Can you work these out from the model? Positions are in its coordinate system, mm. A direction names the side the tool comes from. Give positions to 0.01 mm unless a question says otherwise; leave off trailing zeros. Order: outer loops, then holes, each group sorted by start corner. A loop starts at its lowest first (then second) coordinate and runs counter-clockwise, first axis right, second up. Notation, with made-up numbers: M 23,35.5 L 48,35.5 A23 ccw 48,58.5 Z; hole C -27,9 d7. An arc over 180 degrees is marked long. Answer as a JSON object with one key per item and string values.
```python
from build123d import *

# Parameters (mm, degrees)
SKETCH1_W           = 32
SKETCH1_H           = 22
SKETCH1_W_2         = 30
SKETCH1_H_2         = 20
SKETCH3_W           = 30
SKETCH3_H           = 22
SKETCH3_W_2         = 28
SKETCH3_H_2         = 20
EXTRUDE_THIN1_DEPTH = 150


with BuildPart() as part:
    # Sweep-Thin1: sweep along a path in Sketch2
    with BuildLine(Plane(origin=(0, 0, 0), x_dir=(0, 0, -1), z_dir=(1, 0, 0))) as sweep_thin1_path:
        Line((0, 0), (0, -200))
        Line((0, -200), (428, -200))
        Line((428, -200), (428, 0))
    # Sketch1 → Sweep-Thin1 (sweep)
    with BuildSketch(Plane(origin=(0, 0, 0), x_dir=(1, 0, 0), z_dir=(0, 1, 0))):
        Rectangle(SKETCH1_W, SKETCH1_H)
        Rectangle(SKETCH1_W_2, SKETCH1_H_2, mode=Mode.SUBTRACT)
    sweep_thin1 = sweep(path=sweep_thin1_path.line, transition=Transition.RIGHT)

    # Sketch3 → Extrude-Thin1 (add)
    # profile 1 of 2: a face of its own
    with BuildSketch(Plane(origin=(16, 0, 0), x_dir=(0, 0, -1), z_dir=(1, 0, 0))):
        with Locations((124, -200)):
            Rectangle(SKETCH3_W, SKETCH3_H)
        with Locations((124, -200)):
            Rectangle(SKETCH3_W_2, SKETCH3_H_2, mode=Mode.SUBTRACT)
    # profile 2 of 2: a face of its own
    with BuildSketch(Plane(origin=(16, 0, 0), x_dir=(0, 0, -1), z_dir=(1, 0, 0))):
        with Locations((304, -200)):
            Rectangle(SKETCH3_W, SKETCH3_H)
        with Locations((304, -200)):
            Rectangle(SKETCH3_W_2, SKETCH3_H_2, mode=Mode.SUBTRACT)
    extrude_thin1 = extrude(amount=EXTRUDE_THIN1_DEPTH)

    # Mirror9: Extrude-Thin1 across plane
    add(extrude_thin1.mirror(Plane(origin=(166, 0, 0), x_dir=(0, 0, 1), z_dir=(1, 0, 0))))

    # Mirror10: Sweep-Thin1 across plane
    add(sweep_thin1.mirror(Plane(origin=(166, 0, 0), x_dir=(0, 0, 1), z_dir=(1, 0, 0))))


solid = part.part
```
1) I want a section at C-C on x = 237. Write out the boundary of the cut face in (y, z).
Results found:
{"outline": "M -211,-319 L -189,-319 L -189,-289 L -211,-289 Z; M -211,-139 L -189,-139 L -189,-109 L -211,-109 Z; hole M -210,-318 L -190,-318 L -190,-290 L -210,-290 Z; hole M -210,-138 L -190,-138 L -190,-110 L -210,-110 Z"}
2) Thinking about a two-plate mould opening in X: for faces 1 (the face through (16, -200, -124)), 2 (the face through (331.9, 0, -417.4)), which applies, pulls with the +X half, pulls with the -X half, needs draft (parallel to the pull), parting line crosses it, or undercut?
Results found:
{"face 1": "undercut", "face 2": "needs draft"}
3) I'm going to push flat-ended pins straight in: pin 1 Ø6.5 at (x, y) = (95.5, -205) entering from +Z; pin 2 Ø10 at (x, y) = (115.5, -200) entering from -Z; pin 3 Ø24 at (x, z) = (331.5, -180) entering from +Y. Where does each tip first touch, or does it pass through?
Results found:
{"pin 1": "stops at z = -109", "pin 2": "stops at z = -319", "pin 3": "stops at y = -189"}
4) I need wall thicknesses on L1, parallel to Z at x = 333, y = -157.5; L2, parallel to X at y = -192, z = -66.5; L3, parallel to Y at x = 187, z = -299. Which ranges of each line are inside material? Lowest first, please.
Results found:
{"L1": "z = -439 to -438, -418 to -417, -11 to -10, 10 to 11", "L2": "x = -16 to -15, 15 to 16, 316 to 317, 347 to 348", "L3": "y = -211 to -210, -190 to -189"}
5) I want a section at D-D on z = -302.5. Write out the boundary of the cut face in (x, y).
Results found:
{"outline": "M -16,-211 L 348,-211 L 348,-189 L -16,-189 Z; hole M -15,-210 L 15,-210 L 15,-190 L -15,-190 Z; hole M 16,-210 L 316,-210 L 316,-190 L 16,-190 Z; hole M 317,-210 L 347,-210 L 347,-190 L 317,-190 Z"}
6) I want a section at A-A on y = -180.5. Count the separate pieces of the cut face and the enclosed holes in it, and give its area (3 significant figures).
Results found:
{"separate pieces": "4", "enclosed holes": "4", "area": "416 mm²"}
7) For faces 3 (the face through (16, -137, -419)), 4 (the face through (164, -200, -289)), 5 (the face through (168, -210, -304)), 6 (the face through (168, -200, -109)), 7 (the face through (0, -104, -438)), which set-ups out of +Z, -Z, +X, -X, +Y, -Y let a thin tool reach every point of the face, with its end or its side?
Results found:
{"face 3": "-Z, +Y, -Y", "face 4": "+Y, -Y", "face 5": "none", "face 6": "+Z, +Y, -Y", "face 7": "+Y"}
8) I want a section at B-B on z = -404.5. Write out the boundary of the cut face in (x, y).
Results found:
{"outline": "M -16,-211 L 16,-211 L 16,-189 L -16,-189 Z; M 316,-211 L 348,-211 L 348,-189 L 316,-189 Z; hole M -15,-210 L 15,-210 L 15,-190 L -15,-190 Z; hole M 317,-210 L 347,-210 L 347,-190 L 317,-190 Z"}
